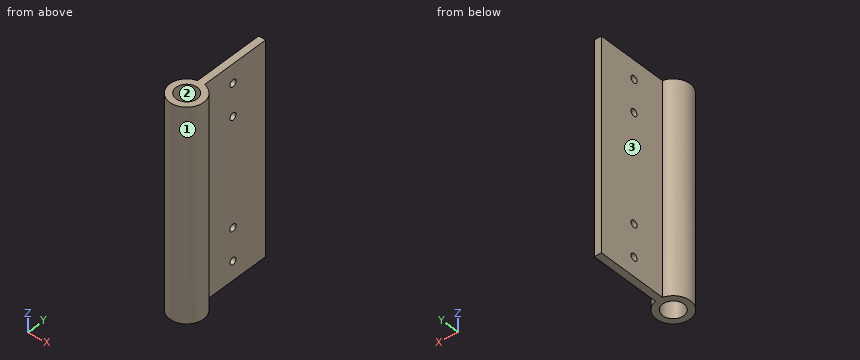
```python
from build123d import *

# Parameters (mm, degrees)
SKETCH1_R           = 7.5
BOSS_EXTRUDE1_DEPTH = 150
SKETCH3_R           = 2.5
CUT_EXTRUDE2_DEPTH  = 163.854749576


with BuildPart() as part:
    # Sketch1 → Boss-Extrude1 (new body)
    with BuildSketch(Plane.XY):
        with BuildLine():
            Line((-2.5, 61.736694594), (-2.5, 11.736694594))
            ThreePointArc((-2.5, 11.736694594), (0, -12), (2.5, 11.736694594))
            Line((2.5, 11.736694594), (2.5, 61.736694594))
            Line((2.5, 61.736694594), (-2.5, 61.736694594))
        make_face()
        Circle(SKETCH1_R, mode=Mode.SUBTRACT)
    extrude(amount=BOSS_EXTRUDE1_DEPTH)

    # Sketch3 → Cut-Extrude2 (cut, through all)
    with BuildSketch(Plane.ZY.offset(2.5)):
        with Locations(Location((113.5, 35, 0), (0, 0, 270))):
            Circle(SKETCH3_R)
        with Locations(Location((136.5, 35, 0), (0, 0, 270))):
            Circle(SKETCH3_R)
        with Locations(Location((36.5, 35, 0), (0, 0, 270))):
            Circle(SKETCH3_R)
        with Locations(Location((13.5, 35, 0), (0, 0, 270))):
            Circle(SKETCH3_R)
    extrude(amount=-CUT_EXTRUDE2_DEPTH, mode=Mode.SUBTRACT)


solid = part.part
```
Check sheet for the modelled part. Datum: model origin and axes. Units: mm. Face numbers are marked on the shaded views. Round coordinates to 2 decimals unless told otherwise and drop trailing zeros. Order: outer loops, then holes, each group sorted by start corner. A loop starts at its lowest first (then second) coordinate and runs counter-clockwise, first axis right, second up. Notation, with made-up numbers: (-25, 69) - (33, 69) arc R13 cw to (33, 75) - close; hole circle Ø9 at (-5.5, -24.5). An arc over 180 degrees is marked (long way). Answer as CSV lines item,"result". Start each with the question number.
1) Draft check along Y on the marked faces 1, 2 and 3. Enter one of: +Y half, -Y half, draft (parallel to the pull), parting line (faces both ways), or undercut.
2) Scan lines: probe 1 along Z at (x, y) = (-0.5, 35); probe 2 along Y at (x, z) = (0, 105); probe 3 along X at (y, z) = (-0.5, 126.5). Record each from-to range of solid material in increasing order.
3) Section check D-D (z = 56). Record the cut outline in (x, y).
4) Section check C-C (y = 35). Record the cut outline in (x, z), then the cut area to 3 significant figures.
5) Section check A-A (x = 0). Record the cut outline in (y, z), then the cut area to 3 significant figures.
6) Depth check by flat-ended pin: pin 1 (6 mm diameter, centred on x = -8, z = 61.5, fed in from +Y); pin 2 (25 mm diameter, centred on y = 42, z = 86, fed in from -X); pin 3 (6 mm diameter, centred on y = 35, z = 136.5, fed in from +X); pin 4 (4.5 mm diameter, centred on y = 35, z = 113.5, fed in from -X). Enter the tip coordinate at first touch or a pass-through.
7) Section check B-B (z = 13.5). Record the cut outline in (x, y), then the cut area to 3 significant figures.
Determined:
1,face 1,"parting line"
1,face 2,"undercut"
1,face 3,"draft"
2,probe 1,"0 to 11, 16 to 34, 39 to 111, 116 to 134, 139 to 150"
2,probe 2,"-12 to -7.5, 7.5 to 61.74"
2,probe 3,"-11.99 to -7.48, 7.48 to 11.99"
3,outline,"(-2.5, 11.74) arc R12 ccw (long way) to (2.5, 11.74) - (2.5, 61.74) - (-2.5, 61.74) - close; hole circle Ø15 at (0, 0)"
4,outline,"(-2.5, 0) - (2.5, 0) - (2.5, 11) - (-2.5, 11) - close; (-2.5, 16) - (2.5, 16) - (2.5, 34) - (-2.5, 34) - close; (-2.5, 39) - (2.5, 39) - (2.5, 111) - (-2.5, 111) - close; (-2.5, 116) - (2.5, 116) - (2.5, 134) - (-2.5, 134) - close; (-2.5, 139) - (2.5, 139) - (2.5, 150) - (-2.5, 150) - close"
4,area,"650 mm^2"
5,outline,"(-12, 0) - (-7.5, 0) - (-7.5, 150) - (-12, 150) - close; (7.5, 0) - (61.74, 0) - (61.74, 150) - (7.5, 150) - close; hole circle Ø5 at (35, 13.5); hole circle Ø5 at (35, 36.5); hole circle Ø5 at (35, 113.5); hole circle Ø5 at (35, 136.5)"
5,area,"8,730 mm^2"
6,pin 1,"y = 10.91"
6,pin 2,"x = -2.5"
6,pin 3,"x = 2.5"
6,pin 4,"through"
7,outline,"(-2.5, 11.74) arc R12 ccw (long way) to (2.5, 11.74) - (2.5, 32.5) - (-2.5, 32.5) - close; (-2.5, 37.5) - (2.5, 37.5) - (2.5, 61.74) - (-2.5, 61.74) - close; hole circle Ø15 at (0, 0)"
7,area,"500 mm^2"
